from build123d import *

# Parameters (mm, degrees)
SKETCH1_W           = 79.5
SKETCH1_H           = 31
BOSS_EXTRUDE1_DEPTH = 12
FILLET1_R           = 2
SHELL1_START        = -37.75
SHELL1_OUTLINE_W    = 8
SHELL1_OUTLINE_H    = 27
SHELL1_DEPTH        = 75.5


# Read off the part's stored shape, not the designer's step: Shell1
with BuildPart() as part:
    # Sketch1 → Boss-Extrude1 (new body)
    with BuildSketch(Plane(origin=(0, 0, 0), x_dir=(1, 0, 0), z_dir=(0, 1, 0))):
        Rectangle(SKETCH1_W, SKETCH1_H)
    extrude(amount=BOSS_EXTRUDE1_DEPTH)

    # Fillet1
    fillet1_edges = [part.edges().sort_by_distance(p)[0] for p in [
        (-39.75, 6, -15.5),
        (39.75, 6, -15.5),
        (39.75, 6, 15.5),
        (-39.75, 6, 15.5),
    ]]
    fillet(fillet1_edges, radius=FILLET1_R)

    # Shell1 outline → Shell1 (cut)
    with BuildSketch(Plane.YZ.offset(SHELL1_START)):
        with Locations((6, 0)):
            Rectangle(SHELL1_OUTLINE_W, SHELL1_OUTLINE_H)
    extrude(amount=SHELL1_DEPTH, mode=Mode.SUBTRACT)


solid = part.part
Geometry check sheet. Reference: the model listing, model coordinates, mm. A direction names the side the tool comes from. Give positions to 0.01 mm unless a question says otherwise; leave off trailing zeros. Write each loop counter-clockwise with the first axis right and the second up, starting at its lowest first coordinate (ties: lowest second). Pieces come first, ordered by that corner, then holes. Notation, with made-up numbers: (-12.5, -10.5) - (21.5, -10.5) arc R32 cw to (21.5, 22.5) - close; hole circle Ø2 at (67, 73.25). An arc over 180 degrees is marked (long way). Put each result on its own line as item: value.
1. Thickness scan on line 1 (Y direction, x = 18, z = -13); line 2 (X direction, y = 9.25, z = 8.5); line 3 (Z direction, x = 13, y = 5.75). Record the ranges inside material, lowest first.
Ans:
line 1: y = 0 to 2, 10 to 12
line 2: x = -39.75 to -37.75, 37.75 to 39.75
line 3: z = -15.5 to -13.5, 13.5 to 15.5
2. Draft check along Y on faces 3 (the flat face through (-1, 12, 0)), 4 (the flat face through (37.75, 6, 0)), 5 (the flat face through (-1, 6, 15.5)). Enter one of: +Y half, -Y half, draft (parallel to the pull), parting line (faces both ways), or undercut.
Ans:
face 3: +Y half
face 4: undercut
face 5: draft
3. Sectioned sample at C-C, the plane z = -7. Enter the section's corners in (x, y).
Ans:
outline: (-39.75, 0) - (39.75, 0) - (39.75, 12) - (-39.75, 12) - close; hole (-37.75, 2) - (37.75, 2) - (37.75, 10) - (-37.75, 10) - close
4. Sectioned sample at A-A, the plane x = 5. Enter the section's corners in (y, z).
Ans:
outline: (0, -15.5) - (12, -15.5) - (12, 15.5) - (0, 15.5) - close; hole (2, -13.5) - (10, -13.5) - (10, 13.5) - (2, 13.5) - close
5. Set-up check for faces 1 (the flat face through (-1, 6, 13.5)), 2 (the flat face through (39.75, 6, 0)): record each of +Z, -Z, +X, -X, +Y, -Y from which the full face is reachable in a straight line by a thin tool's end or side.
Ans:
face 1: none
face 2: +Z, -Z, +X, +Y, -Y
6. Sectioned sample at B-B, the plane y = 4. Enter the section's corners in (x, z), plus the area to 3 significant figures.
Ans:
outline: (-39.75, -13.5) arc R2 ccw to (-37.75, -15.5) - (37.75, -15.5) arc R2 ccw to (39.75, -13.5) - (39.75, 13.5) arc R2 ccw to (37.75, 15.5) - (-37.75, 15.5) arc R2 ccw to (-39.75, 13.5) - close; hole (-37.75, -13.5) - (37.75, -13.5) - (37.75, 13.5) - (-37.75, 13.5) - close
area: 423 mm²
